from build123d import *

# Parameters (mm, degrees)
ESQUISSE1_R        = 1.5
BOSS_EXTRU_1_DEPTH = 26
ESQUISSE2_R        = 2
BOSS_EXTRU_2_DEPTH = 0.5
BOSS_EXTRU_4_START = 0.5
ESQUISSE4_R        = 2
BOSS_EXTRU_4_DEPTH = 0.5


with BuildPart() as part:
    # Esquisse1 → Boss.-Extru.1 (new body)
    with BuildSketch(Plane.XY):
        with Locations(Location((0, 0, 0), (0, 0, 180))):
            Circle(ESQUISSE1_R)
    extrude(amount=BOSS_EXTRU_1_DEPTH)

    # Esquisse2 → Boss.-Extru.2 (add)
    with BuildSketch(Plane.XY.offset(26)):
        Circle(ESQUISSE2_R)
    extrude(amount=BOSS_EXTRU_2_DEPTH)

    # Esquisse4 → Boss.-Extru.4 (add)
    with BuildSketch(Plane(origin=(0, 0, 0), x_dir=(-1, 0, 0), z_dir=(0, 0, -1)).offset(BOSS_EXTRU_4_START)):
        with Locations(Location((0, 0, 0), (0, 0, 180))):
            Circle(ESQUISSE4_R)
    extrude(amount=-BOSS_EXTRU_4_DEPTH)


solid = part.part
Could you check a few things on this model? Use its own coordinates, in mm. Give positions to 0.01 mm unless a question says otherwise; leave off trailing zeros. Order: outer loops, then holes, each group sorted by start corner. A loop starts at its lowest first (then second) coordinate and runs counter-clockwise, first axis right, second up. Notation, with made-up numbers: (-24, 24.25) -> (-19, 24.25) arc R35 ccw to (-19, 63.25) -> close; hole circle Ø10 at (-9.75, 89.5). An arc over 180 degrees is marked (long way). Return JSON: item names as keys, results as strings.
1. Thinking about a two-plate mould opening in Z: for faces 1 (the cylindrical face through (-0.434, 1.952, -0.254)), 2 (the flat face through (0, 0, -0.5)), 3 (the cylindrical face through (-1.43, -0.45, 12.82)), which applies, pulls with the +Z half, pulls with the -Z half, needs draft (parallel to the pull), parting line crosses it, or undercut?
Answer list:
{"face 1": "needs draft", "face 2": "pulls with the -Z half", "face 3": "undercut"}
2. Imagine slicing it at A-A on y = 0. List the corners of the cut face in (x, z) for me, then the cut area to 3 significant figures.
Answer list:
{"outline": "(-2, -0.5) -> (2, -0.5) -> (2, 0) -> (1.5, 0) -> (1.5, 26) -> (2, 26) -> (2, 26.5) -> (-2, 26.5) -> (-2, 26) -> (-1.5, 26) -> (-1.5, 0) -> (-2, 0) -> close", "area": "82.0 mm2"}
3. Imagine slicing it at C-C on z = 15. List the corners of the cut face in (x, y) for me.
Answer list:
{"outline": "circle Ø3 at (0, 0)"}
4. I need wall thicknesses on line 1 (Z direction, x = -1.6, y = -0.2); line 2 (X direction, y = -0.1, z = 6.5); line 3 (Y direction, x = -0.15, z = 16.25). Which ranges of each line are inside material? Lowest first, please. Write a range as from..to.
Answer list:
{"line 1": "z = -0.5..0, 26..26.5", "line 2": "x = -1.5..1.5", "line 3": "y = -1.49..1.49"}
5. For pin 1 Ø2 at (x, z) = (0, 21.5) entering from -Y; pin 2 Ø2 at (x, z) = (-1, 6.5) entering from +Y, each with a flat end and sliding along its axis, tell me the tip position at first contact or that it passes through.
Answer list:
{"pin 1": "stops at y = -1.5", "pin 2": "stops at y = 1.5"}
